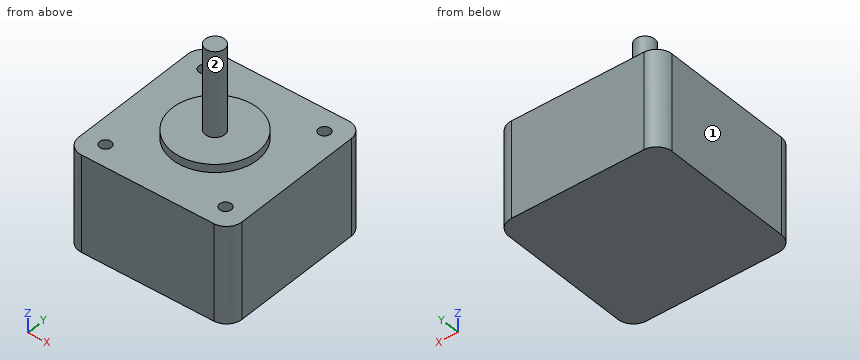
```python
from build123d import *

# Parameters (mm, degrees)
SKIZZE1_W                       = 42.2
SKIZZE1_H                       = 42.2
AUFSATZ_LINEAR_AUSTRAGEN1_DEPTH = 25
SKIZZE2_R                       = 11
AUFSATZ_LINEAR_AUSTRAGEN2_DEPTH = 2.1
SKIZZE3_R                       = 2.5
AUFSATZ_LINEAR_AUSTRAGEN3_DEPTH = 22
SKIZZE4_R                       = 1.5
SCHNITT_LINEAR_AUSTRAGEN1_DEPTH = 4
FILLET1_R                       = 4


with BuildPart() as part:
    # Skizze1 → Aufsatz-Linear austragen1 (new body)
    with BuildSketch(Plane.XY):
        Rectangle(SKIZZE1_W, SKIZZE1_H)
    extrude(amount=AUFSATZ_LINEAR_AUSTRAGEN1_DEPTH)

    # Skizze2 → Aufsatz-Linear austragen2 (add)
    with BuildSketch(Plane.XY.offset(25)):
        Circle(SKIZZE2_R)
    extrude(amount=AUFSATZ_LINEAR_AUSTRAGEN2_DEPTH)

    # Skizze3 → Aufsatz-Linear austragen3 (add)
    with BuildSketch(Plane.XY.offset(27.1)):
        Circle(SKIZZE3_R)
    extrude(amount=AUFSATZ_LINEAR_AUSTRAGEN3_DEPTH)

    # Skizze4 → Schnitt-Linear austragen1 (cut)
    with BuildSketch(Plane.XY.offset(25)):
        with Locations((-15.5, 15.5)):
            Circle(SKIZZE4_R)
        with Locations((15.5, 15.5)):
            Circle(SKIZZE4_R)
        with Locations((15.5, -15.5)):
            Circle(SKIZZE4_R)
        with Locations((-15.5, -15.5)):
            Circle(SKIZZE4_R)
    extrude(amount=-SCHNITT_LINEAR_AUSTRAGEN1_DEPTH, mode=Mode.SUBTRACT)

    # Fillet1
    fillet1_edges = [part.edges().sort_by_distance(p)[0] for p in [
        (21.1, -21.1, 12.5),
        (-21.1, -21.1, 12.5),
        (-21.1, 21.1, 12.5),
        (21.1, 21.1, 12.5),
    ]]
    fillet(fillet1_edges, radius=FILLET1_R)


solid = part.part
```
The listing builds one solid part. Answer for the finished solid, in the listing's coordinates (mm). Face numbers are marked on the shaded views. A direction names the side the tool comes from. Coordinates: 2 decimals unless noted, no trailing zeros. Write each loop counter-clockwise with the first axis right and the second up, starting at its lowest first coordinate (ties: lowest second). Pieces come first, ordered by that corner, then holes. Notation, with made-up numbers: (37, 50.25) - (72, 50.25) arc R24 cw to (72, 68.25) - close; hole circle Ø11 at (-4.5, 33.25). An arc over 180 degrees is marked (long way). One line per item, written item: value.
1) Find section C-C (z = 33.5). Give the vertices of the cut face in (x, y).
Geometry check:
outline: circle Ø5 at (0, 0)
2) Each of these flat-tipped pins is pushed along its axis until it touches: pin 1 Ø2.5 at (x, y) = (-15, -15.5) entering from +Z; pin 2 Ø2.5 at (x, y) = (-15.5, -15.5) entering from +Z; pin 3 Ø6 at (x, z) = (-2, 43) entering from -Y. Where does it stop, or does it pass through?
Geometry check:
pin 1: stops at z = 25
pin 2: stops at z = 21
pin 3: stops at y = -2.5
3) Consider line 1 along Y through (x, z) = (-15.5, 23.95); line 2 along X through (y, z) = (-15, 23); line 3 along Z through (x, y) = (11, -7). Determine where each line is inside the solid, lowest interval first. Write a range as from..to.
Geometry check:
line 1: y = -21.1..-17, -14..14, 17..21.1
line 2: x = -21.1..-16.91, -14.09..14.09, 16.91..21.1
line 3: z = 0..25
4) Find section D-D (y = -5). Give the vertices of the cut face in (x, z).
Geometry check:
outline: (-21.1, 0) - (21.1, 0) - (21.1, 25) - (9.8, 25) - (9.8, 27.1) - (-9.8, 27.1) - (-9.8, 25) - (-21.1, 25) - close
5) Find section B-B (x = 0). Give the vertices of the cut face in (y, z).
Geometry check:
outline: (-21.1, 0) - (21.1, 0) - (21.1, 25) - (11, 25) - (11, 27.1) - (2.5, 27.1) - (2.5, 49.1) - (-2.5, 49.1) - (-2.5, 27.1) - (-11, 27.1) - (-11, 25) - (-21.1, 25) - close
6) A tool of negligible diameter and unlimited length cuts with its end or side. For the marked faces 1 and 2, from which of +Z, -Z, +X, -X, +Y, -Y can it reach the whole face along a straight path? Write none if from no direction.
Geometry check:
face 1: +Z, -Z, -X, +Y, -Y
face 2: +Z
7) Find section A-A (y = 15.5). Give the vertices of the cut face in (x, z).
Geometry check:
outline: (-21.1, 0) - (21.1, 0) - (21.1, 25) - (17, 25) - (17, 21) - (14, 21) - (14, 25) - (-14, 25) - (-14, 21) - (-17, 21) - (-17, 25) - (-21.1, 25) - close
